Drawing for the job (mm, zero at the part's lowest x, y, z). A direction names the side the tool comes from. Give positions to 0.01 mm unless a question says otherwise; leave off trailing zeros. Write each loop counter-clockwise with the first axis right and the second up, starting at its lowest first coordinate (ties: lowest second). Pieces come first, ordered by that corner, then holes. Notation, with made-up numbers: M 79,9 L 100,9 A23 ccw 100,28 Z; hole C -38.75,66 d2. An arc over 180 degrees is marked long. Write item = value, one per line. Start each with the question number.
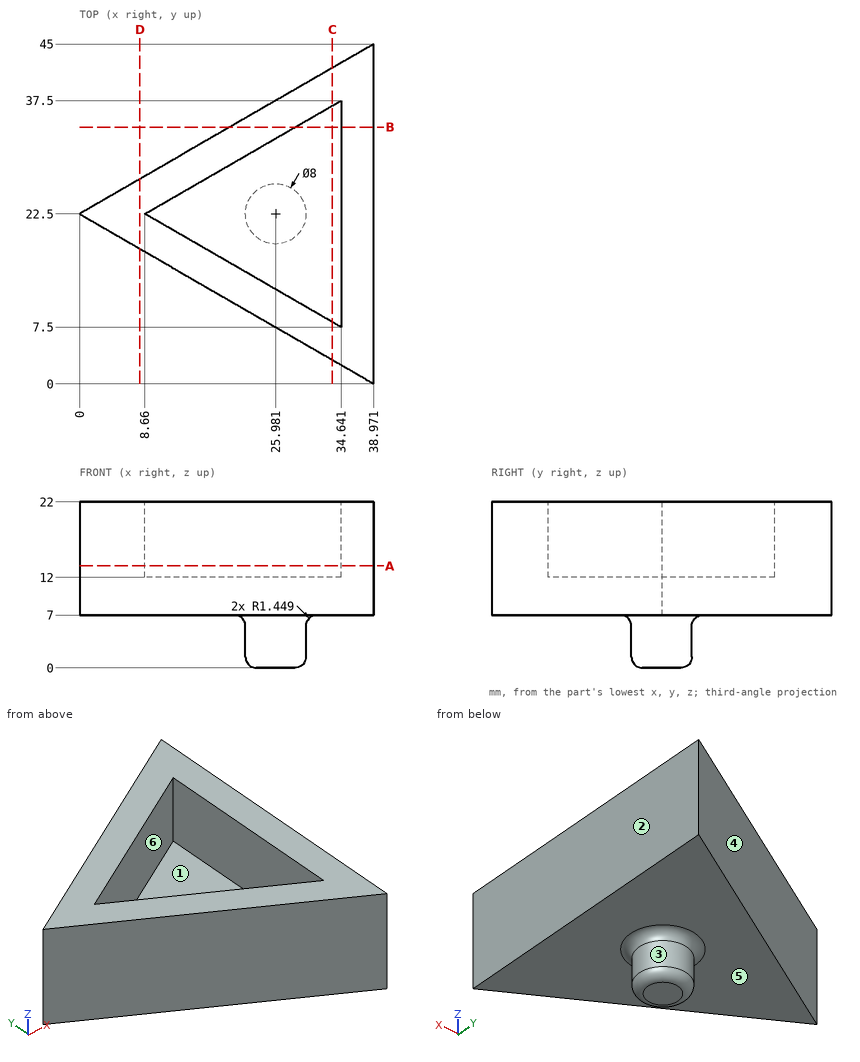
Q1. Drop flat-ended pins along their axis: P1, Ø6, axis at y = 7, z = 15.5, coming from the -X side; P2, Ø10, axis at y = 6, z = 6, coming from the -X side (1 decimal); P3, Ø6, axis at x = 29.5, z = 15, coming from the +Y side (1 decimal); P4, Ø8, axis at x = 12.5, y = 35, coming from the +Z side. Give the stop position or say it passes through.
Q2. Probe line 1 along Z through (x, y) = (37.5, 8); line 2 along X through (y, z) = (18, 12.25) (1 decimal); line 3 along Y through (x, z) = (11, 18.75). List the from-to ranges inside material, lowest first.
Q3. Slice it at A-A (z = 13.5). Give the cut face in (x, y), and give its area (3 significant figures).
Q4. Tool access for the marked faces 1 and 2: list every direction of +Z, -Z, +X, -X, +Y, -Y with a clear straight run to the whole face (end or side of a thin tool).
Q5. Slice it at B-B (y = 34). Give the cut face in (x, z).
Q6. Slice it at C-C (x = 33.5). Give the cut face in (y, z).
Q7. Slice it at D-D (x = 8). Give the cut face in (y, z).
Q8. Two-plate mould, pull along Y, no slides. Class the marked faces 3, 4, 5 and 6: +Y half, -Y half, draft (parallel to the pull), parting line (faces both ways), or undercut.
Working result:
q1.P1 = 21.65
q1.P2 = 20.1
q1.P3 = 41.3
q1.P4 = through
q2.line_1 = 7 to 22
q2.line_2 = 7.8 to 16.5, 34.6 to 39
q2.line_3 = 16.15 to 21.15, 23.85 to 28.85
q3.outline = M 0,22.5 L 38.97,0 L 38.97,45 Z; hole M 8.66,22.5 L 34.64,7.5 L 34.64,37.5 Z
q3.area = 487 mm2
q4.face_1 = +Z
q4.face_2 = +Z, -Z, +X, +Y, -Y
q5.outline = M 19.92,7 L 38.97,7 L 38.97,22 L 34.64,22 L 34.64,12 L 28.58,12 L 28.58,22 L 19.92,22 Z
q6.outline = M 3.16,7 L 41.84,7 L 41.84,22 L 36.84,22 L 36.84,12 L 8.16,12 L 8.16,22 L 3.16,22 Z
q7.outline = M 17.88,7 L 27.12,7 L 27.12,22 L 17.88,22 Z
q8.face_3 = parting line
q8.face_4 = +Y half
q8.face_5 = draft
q8.face_6 = undercut
